Source: CAD feature listing. Evaluate the final solid. Frame: model axes, mm. A direction names the side the tool comes from. Round coordinates to 2 decimals unless told otherwise and drop trailing zeros. Order: outer loops, then holes, each group sorted by start corner. A loop starts at its lowest first (then second) coordinate and runs counter-clockwise, first axis right, second up. Notation, with made-up numbers: (54.25, 14.5) - (86.25, 14.5) arc R21 ccw to (86.25, 41.5) - close; hole circle Ø6 at (-23.5, 57.5). An arc over 180 degrees is marked (long way). Return JSON: item names as keys, results as strings. Group by question number.
1) Section A-A, the plane z = 38.5. Return loops of the section in (x, y), plus the area to 3 significant figures.
2) Ray query, line 1 (Y direction, x = 56, z = 36); line 2 (Z direction, x = 44.5, y = 3). Return the intervals inside material, ascending. Write a range as from..to.
3) Mould query, pull axis X, two halves, no side actions, for faces 1 (the flat face through (30, 58, 59.5)), 2 (the flat face through (2, 30, 0.5)). Classes: pulls with the +X half, pulls with the -X half, needs draft (parallel to the pull), parting line crosses it, or undercut.
4) Section B-B, the plane y = 47. Return loops of the section in (x, z), plus the area to 3 significant figures.
5) Access query for faces 3 (the flat face through (30, 3, 59.5)), 4 (the flat face through (30, 55, 3)), 5 (the flat face through (55, 2, 30)). Directions: +Z, -Z, +X, -X, +Y, -Y. A direction counts if a zero-diameter tool reaches every point of the face in a straight line with its end or side. Return the directions, or none.
6) Contact query for flat-ended pins moving along their axis: P1, Ø12, axis at x = 33, y = 52.5, coming from the +Z side; P2, Ø4, axis at x = 2, y = 26.5, coming from the -Z side. Output: stop coordinate, or through.
```python
from build123d import *

# Parameters (mm, degrees)
F0_W     = 50
F0_H     = 50
F1_DEPTH = 60
F3_DEPTH = 60
F2_W     = 50
F2_H     = 50
F2_H_2   = 19.5
F2_H_3   = 0.5
F2_H_4   = 15
F4_DEPTH = 60
F6_W     = 50
F6_H     = 50
F7_DEPTH = 60


with BuildPart() as f1:
    # F0 (on Right) → F1 (new body)
    with BuildSketch(Plane.YZ):
        Polygon((55, 59.5), (5, 59.5), (5, 60), (0, 60), (0, 0), (5, 0), (5, 0.5), (55, 0.5), (55, 0), (60, 0), (60, 60), (55, 60), align=None)
        with Locations((30, 30)):
            Rectangle(F0_W, F0_H, mode=Mode.SUBTRACT)
    extrude(amount=F1_DEPTH)

    # F0 (on Right) → F3 (join)
    with BuildSketch(Plane.YZ):
        Polygon((55, 59.5), (5, 59.5), (5, 60), (0, 60), (0, 0), (5, 0), (5, 0.5), (55, 0.5), (55, 0), (60, 0), (60, 60), (55, 60), align=None)
        with Locations((30, 30)):
            Rectangle(F0_W, F0_H, mode=Mode.SUBTRACT)
    extrude(amount=F3_DEPTH)

    # F2 (on face) → F4 (cut)
    with BuildSketch(Plane.XZ):
        with Locations((30, 30)):
            Rectangle(F2_W, F2_H)
        with Locations((30, -9.75)):
            Rectangle(F2_W, F2_H_2)
        with Locations((30, 59.75)):
            Rectangle(F2_W, F2_H_3)
        with Locations((30, 0.25)):
            Rectangle(F2_W, F2_H_3)
        with Locations((30, 67.5)):
            Rectangle(F2_W, F2_H_4)
    extrude(amount=-F4_DEPTH, mode=Mode.SUBTRACT)

    # F6 (on offset) → F7 (cut)
    with BuildSketch(Plane.XY.offset(60)):
        with Locations((30, 30)):
            Rectangle(F6_W, F6_H)
    extrude(amount=-F7_DEPTH, mode=Mode.SUBTRACT)


solid = f1.part
```
Geometry check:
{
 "1": {"outline": "(0, 0) - (5, 0) - (5, 5) - (0, 5) - close; (0, 55) - (5, 55) - (5, 60) - (0, 60) - close; (55, 0) - (60, 0) - (60, 5) - (55, 5) - close; (55, 55) - (60, 55) - (60, 60) - (55, 60) - close", "area": "100 mm2"},
 "2": {"line 1": "0..5, 55..60", "line 2": "0.5..5, 55..59.5"},
 "3": {"face 1": "undercut", "face 2": "needs draft"},
 "4": {"outline": "(0, 0.5) - (5, 0.5) - (5, 5) - (0, 5) - close; (0, 55) - (5, 55) - (5, 59.5) - (0, 59.5) - close; (55, 0.5) - (60, 0.5) - (60, 5) - (55, 5) - close; (55, 55) - (60, 55) - (60, 59.5) - (55, 59.5) - close", "area": "90.0 mm2"},
 "5": {"face 3": "+Z, +Y, -Y", "face 4": "+Z, -Z", "face 5": "+Y, -Y"},
 "6": {"P1": "z = 59.5", "P2": "z = 0.5"}
}
